```python
from build123d import *

# Parameters (mm, degrees)
SKETCH1_W           = 1115
SKETCH1_H           = 183
BOSS_EXTRUDE1_DEPTH = 33.45
BOSS_EXTRUDE2_DEPTH = 1115


with BuildPart() as part:
    # Sketch1 → Boss-Extrude1 (new body)
    with BuildSketch(Plane.XY):
        Rectangle(SKETCH1_W, SKETCH1_H)
    extrude(amount=BOSS_EXTRUDE1_DEPTH)

    # Sketch2 → Boss-Extrude2 (add)
    with BuildSketch(Plane(origin=(557.5, 0, 0), x_dir=(0, 0, -1), z_dir=(1, 0, 0))):
        with BuildLine():
            Line((-0.236252667, 159.515154012), (194.779142231, 283.329514055))
            Line((194.779142231, 283.329514055), (212.708104756, 255.090271807))
            Line((212.708104756, 255.090271807), (8.204240057, 125.251726766))
            ThreePointArc((8.204240057, 125.251726766), (5.689681252, 122.973302793), (4.081808438, 119.985165113))
            ThreePointArc((4.081808438, 119.985165113), (0.749606072, 105.927620335), (0, 91.5))
            Line((0, 91.5), (-33.45, 91.5))
            ThreePointArc((-33.45, 91.5), (-25.395939678, 129.684160674), (-0.236252667, 159.515154012))
        make_face()
    extrude(amount=-BOSS_EXTRUDE2_DEPTH)


solid = part.part
```
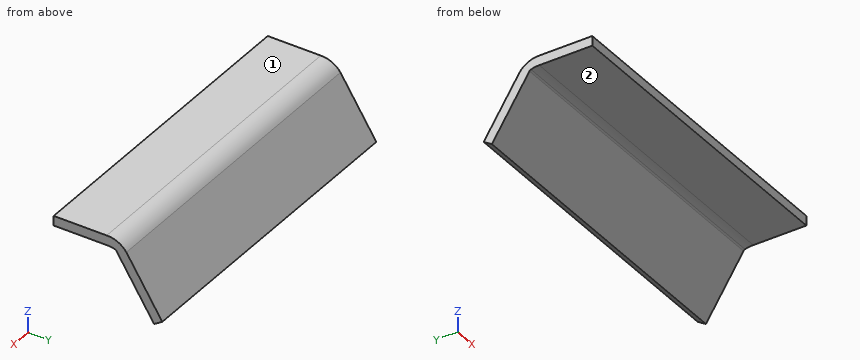
The listing builds one solid part. Answer for the finished solid, in the listing's coordinates (mm). Face numbers are marked on the shaded views. A direction names the side the tool comes from. Give positions to 0.01 mm unless a question says otherwise; leave off trailing zeros. Order: outer loops, then holes, each group sorted by start corner. A loop starts at its lowest first (then second) coordinate and runs counter-clockwise, first axis right, second up. Notation, with made-up numbers: (-33, 21) - (4, 21) arc R18 ccw to (4, 51) - close; hole circle Ø6 at (19.5, 8.5). An arc over 180 degrees is marked (long way). Answer in a Markdown table with one row per item. Add a question column.
Q1. The part is cut by section B-B (y = 42). Determine the outline of the cut face in (x, z), then the cut area to 3 significant figures.
Q2. The part is cut by section A-A (x = -167.5). Determine the outline of the cut face in (y, z).
Q3. Given P1, Ø6, axis at x = 76, z = -118.5, coming from the +Y side; P2, Ø5, axis at x = -375, y = -26.5, coming from the +Z side; P3, Ø1.5, axis at x = -185, z = -110.5, coming from the -Y side, each flat-ended and moving along its own axis, determine where each tip first touches the part or whether it passes through.
Q4. The part is cut by section C-C (z = -100). Determine the outline of the cut face in (x, y).
Q5. Which of the six approach directions +Z, -Z, +X, -X, +Y, -Y give full straight-line access (tool end or side, diameter ignored) to the marked faces 1 and 2?
Q6. Find the intervals of material crossed by line 1 along Z through (x, y) = (132.5, -10); line 2 along Z through (x, y) = (228.5, 123); line 3 along Y through (x, z) = (-59.5, -119.5), in increasing order. Write a range as [from, to].
Determined:
| question | item | result |
|---|---|---|
| 1 | outline | (-557.5, 0) - (557.5, 0) - (557.5, 33.45) - (-557.5, 33.45) - close |
| 1 | area | 37,300 mm² |
| 2 | outline | (-91.5, 0) - (91.5, 0) arc R80 cw to (119.99, -4.08) arc R10 cw to (125.25, -8.2) - (255.09, -212.71) - (283.33, -194.78) - (159.52, 0.24) arc R80 ccw to (91.5, 33.45) - (-91.5, 33.45) - close |
| 3 | P1 | stops at y = 236.8 |
| 3 | P2 | stops at z = 33.45 |
| 3 | P3 | stops at y = 189.72 |
| 4 | outline | (-557.5, 183.53) - (557.5, 183.53) - (557.5, 223.15) - (-557.5, 223.15) - close |
| 5 | face 1 | +Z, +X, -X, +Y, -Y |
| 5 | face 2 | -Z, +X, -X, -Y |
| 6 | line 1 | z = [0, 33.45] |
| 6 | line 2 | z = [-5.71, 28.29] |
| 6 | line 3 | y = [195.91, 235.54] |
